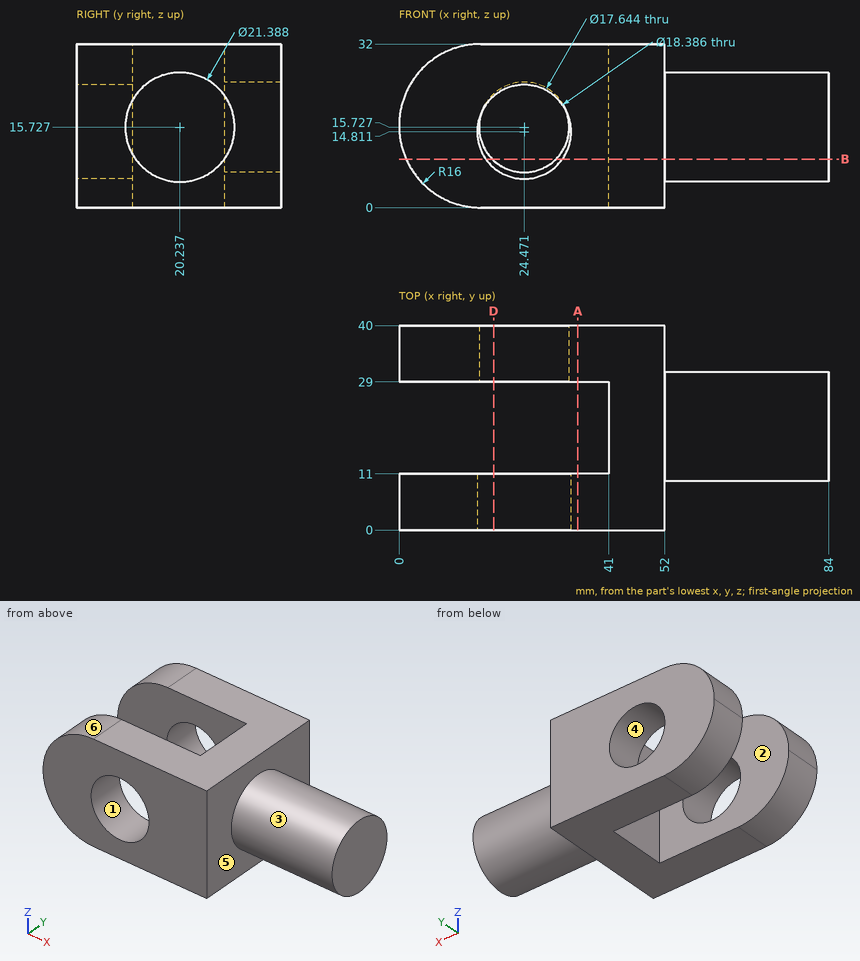
Answer from the drawing. Dimensions are ordinates in mm from the lowest x, y and z of the part. A direction names the side the tool comes from. Coordinates: 2 decimals unless noted, no trailing zeros. Write each loop counter-clockwise with the first axis right and the second up, starting at its lowest first coordinate (ties: lowest second). Pieces come first, ordered by that corner, then holes. Notation, with made-up numbers: (-32, 56.5) - (13, 56.5) arc R31 cw to (13, 88.5) - close; hole circle Ø9 at (19, 6). An arc over 180 degrees is marked (long way). Answer as CSV lines item,"result".
1. Find section A-A (x = 35). Give the vertices of the cut face in (y, z).
Computed values:
outline,"(0, 0) - (11, 0) - (11, 32) - (0, 32) - close; (29, 0) - (40, 0) - (40, 32) - (29, 32) - close"
2. Given P1, Ø4, axis at y = 9, z = 13, coming from the -X side; P2, Ø16, axis at x = 24.47, z = 15.73, coming from the +Y side; P3, Ø2, axis at y = 19.5, z = 13, coming from the -X side; P4, Ø10, axis at x = 71.5, y = 17.5, coming from the -Z side, each flat-ended and moving along its own axis, determine where each tip first touches the part or whether it passes through.
Computed values:
P1,"stops at x = 0.03"
P2,"passes through"
P3,"stops at x = 41"
P4,"stops at z = 5.03"
3. Straight lines are drawn through the part: line 1 (Y direction, x = 7.5, z = 9.5); line 2 (X direction, y = 16.5, z = 20.5); line 3 (Z direction, x = 68.5, y = 20.5). For each, find the intervals that lie inside material, in ascending order. Write a range as [from, to].
Computed values:
line 1,"y = [0, 11], [29, 40]"
line 2,"x = [41, 84]"
line 3,"z = [5.04, 26.42]"
4. Determine the mould class of the marked faces 4, 5 and 6 for opening direction X: +X half, -X half, draft (parallel to the pull), parting line (faces both ways), or undercut.
Computed values:
face 4,"undercut"
face 5,"+X half"
face 6,"-X half"
5. Find section D-D (x = 18.5). Give the vertices of the cut face in (y, z), plus the area to 3 significant figures.
Computed values:
outline,"(0, 0) - (11, 0) - (11, 7.82) - (0, 7.82) - close; (0, 21.8) - (11, 21.8) - (11, 32) - (0, 32) - close; (29, 0) - (40, 0) - (40, 9.23) - (29, 9.23) - close; (29, 22.22) - (40, 22.22) - (40, 32) - (29, 32) - close"
area,"407 mm²"
6. Find section B-B (z = 9.5). Give the vertices of the cut face in (x, y) (1 decimal), plus the area to 3 significant figures.
Computed values:
outline,"(1.4, 0) - (17, 0) - (17, 11) - (1.4, 11) - close; (1.4, 29) - (18.2, 29) - (18.2, 40) - (1.4, 40) - close; (30.7, 29) - (41, 29) - (41, 11) - (32, 11) - (32, 0) - (52, 0) - (52, 11.5) - (84, 11.5) - (84, 28.9) - (52, 28.9) - (52, 40) - (30.7, 40) - close"
area,"1,570 mm²"
7. A tool of negligible diameter and unlimited length cuts with its end or side. For the marked faces 1, 2 and 3, from which of +Z, -Z, +X, -X, +Y, -Y can it reach the whole face along a straight path? Write none if from no direction.
Computed values:
face 1,"-Y"
face 2,"+Z, -Z, -X"
face 3,"+X"
